```python
from build123d import *

# Parameters (mm, degrees)
SKETCH1_R           = 8
BOSS_EXTRUDE1_DEPTH = 20
SKETCH2_W           = 60
SKETCH2_H           = 3
BOSS_EXTRUDE2_DEPTH = 15
SKETCH3_R           = 2.5
CUT_EXTRUDE1_DEPTH  = 20
FILLET1_R           = 5


with BuildPart() as part:
    # Sketch1 → Boss-Extrude1 (new body)
    with BuildSketch(Plane.XY):
        with BuildLine():
            Line((30, -28.5), (30, -38.5))
            Line((30, -38.5), (-30, -38.5))
            Line((-30, -38.5), (-30, -28.5))
            Line((-30, -28.5), (-11.461412637, 6.13482032))
            ThreePointArc((-11.461412637, 6.13482032), (0, 13), (11.461412637, 6.13482032))
            Line((11.461412637, 6.13482032), (30, -28.5))
        make_face()
        Circle(SKETCH1_R, mode=Mode.SUBTRACT)
    extrude(amount=BOSS_EXTRUDE1_DEPTH)

    # Sketch2 → Boss-Extrude2 (add)
    with BuildSketch(Plane(origin=(0, 0, 0), x_dir=(-1, 0, 0), z_dir=(0, 0, -1))):
        with Locations((0, -37)):
            Rectangle(SKETCH2_W, SKETCH2_H)
    extrude(amount=BOSS_EXTRUDE2_DEPTH)

    # Sketch3 → Cut-Extrude1 (cut)
    with BuildSketch(Plane.XZ.offset(38.5)):
        with Locations((22.5, -7.5)):
            Circle(SKETCH3_R)
        with Locations((-22.5, -7.5)):
            Circle(SKETCH3_R)
    extrude(amount=-CUT_EXTRUDE1_DEPTH, mode=Mode.SUBTRACT)

    # Fillet1
    fillet1_edges = [part.edges().sort_by_distance(p)[0] for p in [
        (30, -37, -15),
        (-30, -37, -15),
        (0, -38.5, 20),
    ]]
    fillet(fillet1_edges, radius=FILLET1_R)


solid = part.part
```
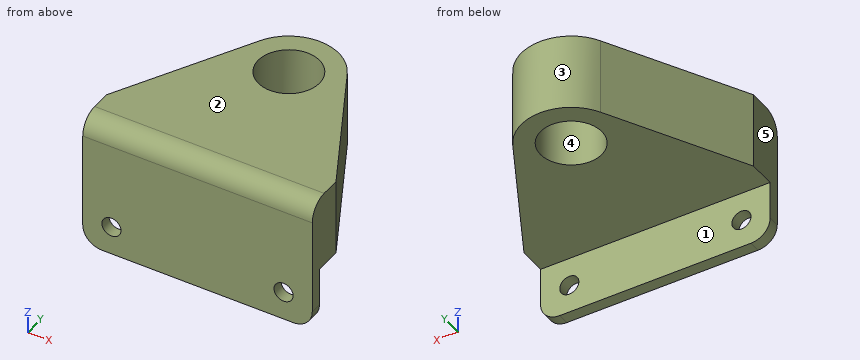
The model under review builds one solid part; all positions refer to its coordinate system, in mm. Face numbers are marked on the shaded views. A direction names the side the tool comes from. Give positions to 0.01 mm unless a question says otherwise; leave off trailing zeros. Write each loop counter-clockwise with the first axis right and the second up, starting at its lowest first coordinate (ties: lowest second). Pieces come first, ordered by that corner, then holes.
(1) For P1, Ø8, axis at x = -16.5, z = 14, coming from the +Y side; P2, Ø10, axis at y = -13, z = 9, coming from the +X side; P3, Ø21, axis at x = 0, y = 0, coming from the -Z side, all flat-tipped, find the tip position at first contact; note any pin that passes through.
(2) Consider section D-D, the plane y = 0. Give the boundary of the cut face in (x, z).
(3) To check wall thickness, follow L1, parallel to Y at x = 0, z = 6.75; L2, parallel to Z at x = -23, y = -33; L3, parallel to Y at x = -1.5, z = 11.5. State the ranges of each line that lie inside material, in increasing order.
(4) The part is to be moulded in two halves that separate along X. For the marked faces 3, 4 and 5, say which applies: released by +X, released by -X, zero draft, split by the parting line, or undercut.
(5) Consider section A-A, the plane z = -7.5. Give the boundary of the cut face in (x, y).
(6) Consider section C-C, the plane z = 1. Give the boundary of the cut face in (x, y), and give its area (3 significant figures).
(7) Consider section B-B, the plane x = 0. Give the boundary of the cut face in (y, z), and give its area (3 significant figures).
(8) Tool access review of the marked faces 1 and 2: name each direction out of +Z, -Z, +X, -X, +Y, -Y from which nothing blocks a thin tool from reaching the whole face with its end or side.
Returned:
1. P1: stops at y = 4.19
1. P2: stops at x = 24.38
1. P3: stops at z = 0
2. outline: (-14.75, 0) - (-8, 0) - (-8, 20) - (-14.75, 20) - close; (8, 0) - (14.75, 0) - (14.75, 20) - (8, 20) - close
3. L1: y = -38.5 to -8, 8 to 13
3. L2: z = 0 to 20
3. L3: y = -38.5 to -7.86, 7.86 to 12.91
4. face 3: split by the parting line
4. face 4: undercut
4. face 5: released by -X
5. outline: (-30, -38.5) - (-25, -38.5) - (-25, -35.5) - (-30, -35.5) - close; (-20, -38.5) - (20, -38.5) - (20, -35.5) - (-20, -35.5) - close; (25, -38.5) - (30, -38.5) - (30, -35.5) - (25, -35.5) - close
6. outline: (-30, -38.5) - (30, -38.5) - (30, -28.5) - (11.46, 6.13) arc R13 ccw to (-11.46, 6.13) - (-30, -28.5) - close; hole circle Ø16 at (0, 0)
6. area: 1,950 mm2
7. outline: (-38.5, -15) - (-35.5, -15) - (-35.5, 0) - (-8, 0) - (-8, 20) - (-33.5, 20) arc R5 ccw to (-38.5, 15) - close; (8, 0) - (13, 0) - (13, 20) - (8, 20) - close
7. area: 750 mm2
8. face 1: -Z, +X, -X, +Y
8. face 2: +Z, +X, -X, +Y, -Y
